Verification items for the finished model (mm, model axes). A direction names the side the tool comes from. Round coordinates to 2 decimals unless told otherwise and drop trailing zeros. Order: outer loops, then holes, each group sorted by start corner. A loop starts at its lowest first (then second) coordinate and runs counter-clockwise, first axis right, second up. Notation, with made-up numbers: (-27.75, 60.25) -> (-14.75, 60.25) arc R29 ccw to (-14.75, 92.25) -> close; hole circle Ø2 at (-36.75, 21.5). An arc over 180 degrees is marked (long way). Return JSON: item names as keys, results as strings. Group by question number.
1) Section check A-A on z = 86.5. Enter the section's corners in (x, y), plus the area to 3 significant figures.
2) Section check B-B on z = 24.5. Enter the section's corners in (x, y).
3) Draft check along Z on faces 1 (the flat face through (-3, 6, 152.4)), 2 (the flat face through (-2.19, -61.99, 1.88)), 3 (the flat face through (-3, 6, 50.8)). Enter one of: pulls with the +Z half, pulls with the -Z half, needs draft (parallel to the pull), parting line crosses it, or undercut.
4) Scan lines: L1, parallel to Z at x = -6, y = 61; L2, parallel to X at y = 2, z = 98.5; L3, parallel to X at y = -1, z = 150. Record each from-to range of solid material in increasing order.
5) Depth check by flat-ended pin: pin 1 (10 mm diameter, centred on x = -38.74, y = -19.61, fed in from +Z); pin 2 (1 mm diameter, centred on x = 5.5, z = 27.5, fed in from -Y). Enter the tip coordinate at first touch or a pass-through.
6) Tool access check on faces 4 (the flat face through (61.4, -16.9, 1.9)), 5 (the flat face through (-7.88, 63.19, 1.88)), 6 (the cylindrical face through (-1.38, -6.2, 165.28)), 7 (the flat face through (-25.747, -56.428, 1.878)). Record the directions out of +Z, -Z, +X, -X, +Y, -Y that give a thin tool (end or side, any length) a straight path to the whole face; none if there is none.
```python
from build123d import *

# Parameters (mm, degrees)
F4_R      = 6.35
F5_DEPTH  = 177.8
F6_R      = 3.175
F7_DEPTH  = 3.81
F9_R      = 7.62
F10_DEPTH = 50.8


with BuildPart() as f5:
    # F4 (on offset) → F5 (new body)
    with BuildSketch(Plane.XY.offset(177.8)):
        Circle(F4_R)
    extrude(amount=-F5_DEPTH)

    # F6 (on Top) → F7 (join)
    with BuildSketch(Plane.XY):
        with BuildLine():
            Line((44.471199, 24.555091), (46.317659, 60.507144))
            Line((46.317659, 60.507144), (31.689204, 39.704337))
            ThreePointArc((31.689204, 39.704337), (38.826236, 32.759172), (44.471199, 24.555091))
        make_face()
        with BuildLine():
            Line((31.689204, 39.704337), (19.636856, 73.626313))
            Line((19.636856, 73.626313), (14.082815, 48.808957))
            ThreePointArc((14.082815, 48.808957), (23.334373, 45.123686), (31.689204, 39.704337))
        make_face()
        with BuildLine():
            Line((14.082815, 48.808957), (-10.033481, 75.536543))
            Line((-10.033481, 75.536543), (-5.667555, 50.482857))
            ThreePointArc((-5.667555, 50.482857), (4.290062, 50.618528), (14.082815, 48.808957))
        make_face()
        with BuildLine():
            Line((-5.667555, 50.482857), (-38.176311, 65.947019))
            Line((-38.176311, 65.947019), (-24.555091, 44.471199))
            ThreePointArc((-24.555091, 44.471199), (-15.407371, 48.407158), (-5.667555, 50.482857))
        make_face()
        with BuildLine():
            Line((-24.555091, 44.471199), (-60.507144, 46.317659))
            Line((-60.507144, 46.317659), (-39.704337, 31.689204))
            ThreePointArc((-39.704337, 31.689204), (-32.759172, 38.826236), (-24.555091, 44.471199))
        make_face()
        with BuildLine():
            Line((-39.704337, 31.689204), (-73.626313, 19.636856))
            Line((-73.626313, 19.636856), (-48.808957, 14.082815))
            ThreePointArc((-48.808957, 14.082815), (-45.123686, 23.334373), (-39.704337, 31.689204))
        make_face()
        with BuildLine():
            Line((-48.808957, 14.082815), (-75.536543, -10.033481))
            Line((-75.536543, -10.033481), (-50.482857, -5.667555))
            ThreePointArc((-50.482857, -5.667555), (-50.618528, 4.290062), (-48.808957, 14.082815))
        make_face()
        with BuildLine():
            Line((-50.482857, -5.667555), (-65.947019, -38.176311))
            Line((-65.947019, -38.176311), (-44.471199, -24.555091))
            ThreePointArc((-44.471199, -24.555091), (-48.407158, -15.407371), (-50.482857, -5.667555))
        make_face()
        with BuildLine():
            Line((-44.471199, -24.555091), (-46.317659, -60.507144))
            Line((-46.317659, -60.507144), (-31.689204, -39.704337))
            ThreePointArc((-31.689204, -39.704337), (-38.826236, -32.759172), (-44.471199, -24.555091))
        make_face()
        with BuildLine():
            Line((50.482857, 5.667555), (65.947019, 38.176311))
            Line((65.947019, 38.176311), (44.471199, 24.555091))
            ThreePointArc((44.471199, 24.555091), (48.407158, 15.407371), (50.482857, 5.667555))
        make_face()
        with BuildLine():
            Line((39.704337, -31.689204), (73.626313, -19.636856))
            Line((73.626313, -19.636856), (48.808957, -14.082815))
            ThreePointArc((48.808957, -14.082815), (45.123686, -23.334373), (39.704337, -31.689204))
        make_face()
        with BuildLine():
            Line((24.555091, -44.471199), (60.507144, -46.317659))
            Line((60.507144, -46.317659), (39.704337, -31.689204))
            ThreePointArc((39.704337, -31.689204), (32.759172, -38.826236), (24.555091, -44.471199))
        make_face()
        with BuildLine():
            Line((5.667555, -50.482857), (38.176311, -65.947019))
            Line((38.176311, -65.947019), (24.555091, -44.471199))
            ThreePointArc((24.555091, -44.471199), (15.407371, -48.407158), (5.667555, -50.482857))
        make_face()
        with BuildLine():
            Line((-31.689204, -39.704337), (-19.636856, -73.626313))
            Line((-19.636856, -73.626313), (-14.082815, -48.808957))
            ThreePointArc((-14.082815, -48.808957), (-23.334373, -45.123686), (-31.689204, -39.704337))
        make_face()
        with BuildLine():
            Line((48.808957, -14.082815), (75.536543, 10.033481))
            Line((75.536543, 10.033481), (50.482857, 5.667555))
            ThreePointArc((50.482857, 5.667555), (50.720652, 2.838211), (50.8, 0))
            ThreePointArc((50.8, 0), (50.299777, -7.111433), (48.808957, -14.082815))
        make_face()
        with BuildLine():
            ThreePointArc((50.8, 0), (50.720652, 2.838211), (50.482857, 5.667555))
            ThreePointArc((50.482857, 5.667555), (48.407158, 15.407371), (44.471199, 24.555091))
            ThreePointArc((44.471199, 24.555091), (38.826236, 32.759172), (31.689204, 39.704337))
            ThreePointArc((31.689204, 39.704337), (23.334373, 45.123686), (14.082815, 48.808957))
            ThreePointArc((14.082815, 48.808957), (4.290062, 50.618528), (-5.667555, 50.482857))
            ThreePointArc((-5.667555, 50.482857), (-15.407371, 48.407158), (-24.555091, 44.471199))
            ThreePointArc((-24.555091, 44.471199), (-32.759172, 38.826236), (-39.704337, 31.689204))
            ThreePointArc((-39.704337, 31.689204), (-45.123686, 23.334373), (-48.808957, 14.082815))
            ThreePointArc((-48.808957, 14.082815), (-50.618528, 4.290062), (-50.482857, -5.667555))
            ThreePointArc((-50.482857, -5.667555), (-48.407158, -15.407371), (-44.471199, -24.555091))
            ThreePointArc((-44.471199, -24.555091), (-38.826236, -32.759172), (-31.689204, -39.704337))
            ThreePointArc((-31.689204, -39.704337), (-23.334373, -45.123686), (-14.082815, -48.808957))
            ThreePointArc((-14.082815, -48.808957), (-4.290062, -50.618528), (5.667555, -50.482857))
            ThreePointArc((5.667555, -50.482857), (15.407371, -48.407158), (24.555091, -44.471199))
            ThreePointArc((24.555091, -44.471199), (32.759172, -38.826236), (39.704337, -31.689204))
            ThreePointArc((39.704337, -31.689204), (45.123686, -23.334373), (48.808957, -14.082815))
            ThreePointArc((48.808957, -14.082815), (50.299777, -7.111433), (50.8, 0))
        make_face()
        with Locations((-13.52704, -41.260585)):
            Circle(F6_R, mode=Mode.SUBTRACT)
        with Locations((-38.740702, -19.610578)):
            Circle(F6_R, mode=Mode.SUBTRACT)
        with Locations((-21.079572, -24.881321)):
            Circle(F6_R, mode=Mode.SUBTRACT)
        with Locations((-32.499259, -2.688243)):
            Circle(F6_R, mode=Mode.SUBTRACT)
        with Locations((-5.250672, -17.614936)):
            Circle(F6_R, mode=Mode.SUBTRACT)
        with Locations((-16.168427, -8.742855)):
            Circle(F6_R, mode=Mode.SUBTRACT)
        with Locations((19.610578, -38.740702)):
            Circle(F6_R, mode=Mode.SUBTRACT)
        with Locations((2.688243, -32.499259)):
            Circle(F6_R, mode=Mode.SUBTRACT)
        with Locations((24.881321, -21.079572)):
            Circle(F6_R, mode=Mode.SUBTRACT)
        with Locations((8.742855, -16.168427)):
            Circle(F6_R, mode=Mode.SUBTRACT)
        with Locations((17.614936, -5.250672)):
            Circle(F6_R, mode=Mode.SUBTRACT)
        with Locations((41.260585, -13.52704)):
            Circle(F6_R, mode=Mode.SUBTRACT)
        with Locations((-41.260585, 13.52704)):
            Circle(F6_R, mode=Mode.SUBTRACT)
        with Locations((-17.614936, 5.250672)):
            Circle(F6_R, mode=Mode.SUBTRACT)
        with Locations((-8.742855, 16.168427)):
            Circle(F6_R, mode=Mode.SUBTRACT)
        with Locations((-24.881321, 21.079572)):
            Circle(F6_R, mode=Mode.SUBTRACT)
        with Locations((-2.688243, 32.499259)):
            Circle(F6_R, mode=Mode.SUBTRACT)
        with Locations((-19.610578, 38.740702)):
            Circle(F6_R, mode=Mode.SUBTRACT)
        with Locations((16.168427, 8.742855)):
            Circle(F6_R, mode=Mode.SUBTRACT)
        with Locations((5.250672, 17.614936)):
            Circle(F6_R, mode=Mode.SUBTRACT)
        with Locations((32.499259, 2.688243)):
            Circle(F6_R, mode=Mode.SUBTRACT)
        with Locations((21.079572, 24.881321)):
            Circle(F6_R, mode=Mode.SUBTRACT)
        with Locations((38.740702, 19.610578)):
            Circle(F6_R, mode=Mode.SUBTRACT)
        with Locations((13.52704, 41.260585)):
            Circle(F6_R, mode=Mode.SUBTRACT)
        with BuildLine():
            Line((-14.082815, -48.808957), (10.033481, -75.536543))
            Line((10.033481, -75.536543), (5.667555, -50.482857))
            ThreePointArc((5.667555, -50.482857), (-4.290062, -50.618528), (-14.082815, -48.808957))
        make_face()
    extrude(amount=F7_DEPTH)

    # F9 (on offset) → F10 (join, symmetric)
    with BuildSketch(Plane.XY.offset(101.6)):
        Circle(F9_R)
    extrude(amount=F10_DEPTH, both=True)


solid = f5.part
```
Check result:
{
 "1": {"outline": "circle Ø15.24 at (0, 0)", "area": "182 mm^2"},
 "2": {"outline": "circle Ø12.7 at (0, 0)"},
 "3": {"face 1": "pulls with the +Z half", "face 2": "needs draft", "face 3": "undercut"},
 "4": {"L1": "0 to 3.81", "L2": "-7.35 to 7.35", "L3": "-7.55 to 7.55"},
 "5": {"pin 1": "z = 3.81", "pin 2": "y = -3.91"},
 "6": {"face 4": "+Z, -Z, +X", "face 5": "+Z, -Z", "face 6": "+Z", "face 7": "+Z, -Z, -Y"}
}
